```python
from build123d import *


with BuildPart() as part:
    # Skizze1 → Rotation1 (revolve)
    with BuildSketch(Plane.XY, mode=Mode.PRIVATE) as rotation1_sk:
        with BuildLine():
            Line((21, 40), (21, 0))
            Line((21, 0), (22.5, 0))
            Line((22.5, 0), (22.5, 30.992047723))
            ThreePointArc((22.5, 30.992047723), (22.750654736, 31.654227211), (23.376963351, 31.98444985))
            ThreePointArc((23.376963351, 31.98444985), (64.24040311, 41.730422057), (101.963350785, 60.217820521))
            ThreePointArc((101.963350785, 60.217820521), (102.981326701, 60.250556357), (103.5, 59.374015081))
            Line((103.5, 59.374015081), (103.5, 0))
            Line((103.5, 0), (105, 0))
            Line((105, 0), (105, 70.490862433))
            ThreePointArc((105, 70.490862433), (103.931735943, 72.260570921), (101.868131868, 72.13976344))
            ThreePointArc((101.868131868, 72.13976344), (64.106096115, 52.343326056), (22.747252747, 41.98396543))
            ThreePointArc((22.747252747, 41.98396543), (21.499084528, 41.321836884), (21, 40))
        make_face()
    revolve(rotation1_sk.sketch.rotate(Axis((0, 0, 0), (0, 1, 0)), 90), axis=Axis((0, 0, 0), (0, 1, 0)))  # turned: the seam where the file's is

    # Skizze3 → Schnitt-Rotation1 (revolve, cut)
    with BuildSketch(Plane.XY):
        Polygon((41.739821974, 45.447201272), (42.516279109, 42.549423793), (45.897019501, 43.455290451), (48.226390907, 34.761958014), (49.675279646, 35.150186582), (46.569451105, 46.741296497), align=None)
    revolve(axis=Axis((0, 220.540854102, 0), (0.258819045, -0.965925826, 0)), mode=Mode.SUBTRACT)


solid = part.part
```
Work out the finished part from the listing and answer in its coordinate system (mm). A direction names the side the tool comes from. Round coordinates to 2 decimals unless told otherwise and drop trailing zeros. Write each loop counter-clockwise with the first axis right and the second up, starting at its lowest first coordinate (ties: lowest second). Pieces come first, ordered by that corner, then holes.
1) Which of the six approach directions +Z, -Z, +X, -X, +Y, -Y give full straight-line access (tool end or side, diameter ignored) to faces 4 (the face through (19.961, 15.713, -10.382)), 5 (the face through (-6.31, 19.72, -20.03))?
2) Determine the mould class of faces 1 (the face through (70, 0, 77)), 2 (the face through (-31.54, 35.74, -100.15)), 3 (the face through (-31.09, 29.27, -98.72)) for opening direction X: pulls with the +X half, pulls with the -X half, needs draft (parallel to the pull), parting line crosses it, or undercut.
3) A cutting plane is placed at C-C on y = 54.5. Determine the outline of the cut face in (x, z), and give its area (3 significant figures).
4) A cutting plane is placed at A-A on x = 0. Determine the outline of the cut face in (y, z), and give its area (3 significant figures).
5) A cutting plane is placed at B-B on y = 7.5. Determine the outline of the cut face in (x, z), and give its area (3 significant figures).
6) Consider probe 1 along X at (y, z) = (22.5, 0); probe 2 along X at (y, z) = (5, -3.5); probe 3 along Z at (x, y) = (-90.5, 19). Determine where each line is inside the solid, lowest interval first.
7) Flat-ended cylindrical pins translate along their axes: P1, Ø1, axis at x = 22, z = 27, coming from the +Y side; P2, Ø8, axis at x = 49, y = 33, coming from the -Z side; P3, Ø8, axis at x = 50.5, z = -12, coming from the -Y side; P4, Ø25, axis at x = 0, z = 0, coming from the -Y side. Find the tip coordinate at first contact, or state that the pin passes through.
Entries:
1. face 4: -Y
1. face 5: +Y, -Y
2. face 1: needs draft
2. face 2: parting line crosses it
2. face 3: undercut
3. outline: circle Ø210 at (0, 0); circle Ø184.72 at (0, 0); hole circle Ø207 at (0, 0); hole circle Ø139 at (0, 0)
3. area: 12,600 mm2
4. outline: (0, -105) - (70.49, -105) arc R2 ccw to (72.14, -101.87) arc R180 cw to (41.98, -22.75) arc R2 ccw to (40, -21) - (0, -21) - (0, -22.5) - (30.99, -22.5) arc R1 cw to (31.98, -23.38) arc R190 ccw to (60.22, -101.96) arc R1 cw to (59.37, -103.5) - (0, -103.5) - close; (0, 21) - (40, 21) arc R2 ccw to (41.98, 22.75) arc R180 cw to (72.14, 101.87) arc R2 ccw to (70.49, 105) - (0, 105) - (0, 103.5) - (59.37, 103.5) arc R1 cw to (60.22, 101.96) arc R190 ccw to (31.98, 23.38) arc R1 cw to (30.99, 22.5) - (0, 22.5) - close
4. area: 2,090 mm2
5. outline: circle Ø210 at (0, 0); circle Ø45 at (0, 0); hole circle Ø207 at (0, 0); hole circle Ø42 at (0, 0)
5. area: 1,190 mm2
6. probe 1: x = -105 to -103.5, -22.5 to -21, 21 to 22.5, 103.5 to 105
6. probe 2: x = -104.94 to -103.44, -22.23 to -20.71, 20.71 to 22.23, 103.44 to 104.94
6. probe 3: z = -53.24 to -50.22, 50.22 to 53.24
7. P1: stops at y = 44.04
7. P2: stops at z = -94.87
7. P3: stops at y = 36.68
7. P4: passes through
